Answer from the drawing. Dimensions are ordinates in mm from the lowest x, y and z of the part. Coordinates: 2 decimals unless noted, no trailing zeros. Write each loop counter-clockwise with the first axis right and the second up, starting at its lowest first coordinate (ties: lowest second). Pieces come first, ordered by that corner, then holes.
1) The part is cut by section D-D (z = 14.5). Determine the outline of the cut face in (x, y).
2) Each of these flat-tipped pins is pushed along its axis until it touches: pin 1 Ø1.5 at (x, y) = (70, 1) entering from -Z; pin 2 Ø0.9 at (x, y) = (3, 1) entering from +Z; pin 3 Ø0.9 at (y, z) = (1.5, 36.5) entering from -X; pin 4 Ø12 at (x, z) = (34, 14) entering from +Y. Where does it stop, or does it pass through?
3) The part is cut by section A-A (z = 24). Determine the outline of the cut face in (x, y).
4) The part is cut by section C-C (y = 2.05). Determine the outline of the cut face in (x, z), then the cut area to 3 significant figures.
5) Find the intervals of material crossed by line 1 (X direction, y = 1.7, z = 29); line 2 (X direction, y = 0.2, z = 15); line 3 (Z direction, x = 41.5, y = 2.25), in increasing order.
6) The part is cut by section B-B (x = 26.5). Determine the outline of the cut face in (y, z).
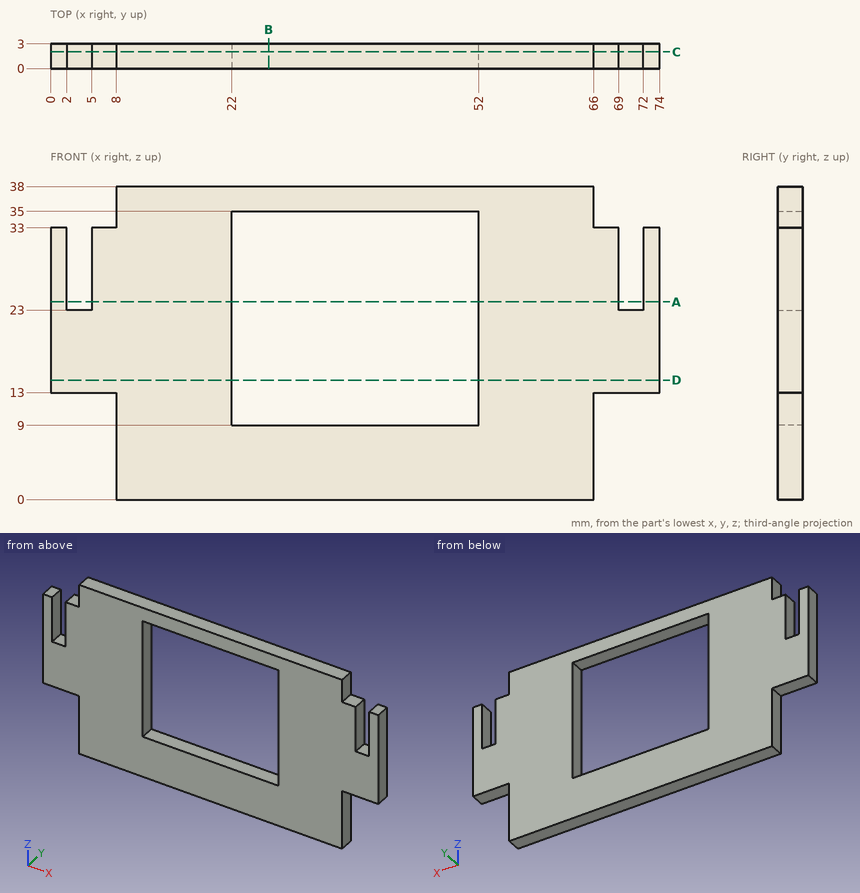
Reported:
1. outline: (0, 0) - (22, 0) - (22, 3) - (0, 3) - close; (52, 0) - (74, 0) - (74, 3) - (52, 3) - close
2. pin 1: stops at z = 13
2. pin 2: stops at z = 23
2. pin 3: stops at x = 8
2. pin 4: stops at y = 3
3. outline: (0, 0) - (2, 0) - (2, 3) - (0, 3) - close; (5, 0) - (22, 0) - (22, 3) - (5, 3) - close; (52, 0) - (69, 0) - (69, 3) - (52, 3) - close; (72, 0) - (74, 0) - (74, 3) - (72, 3) - close
4. outline: (0, 13) - (8, 13) - (8, 0) - (66, 0) - (66, 13) - (74, 13) - (74, 33) - (72, 33) - (72, 23) - (69, 23) - (69, 33) - (66, 33) - (66, 38) - (8, 38) - (8, 33) - (5, 33) - (5, 23) - (2, 23) - (2, 33) - (0, 33) - close; hole (22, 9) - (52, 9) - (52, 35) - (22, 35) - close
4. area: 1,680 mm2
5. line 1: x = 0 to 2, 5 to 22, 52 to 69, 72 to 74
5. line 2: x = 0 to 22, 52 to 74
5. line 3: z = 0 to 9, 35 to 38
6. outline: (0, 0) - (3, 0) - (3, 9) - (0, 9) - close; (0, 35) - (3, 35) - (3, 38) - (0, 38) - close
